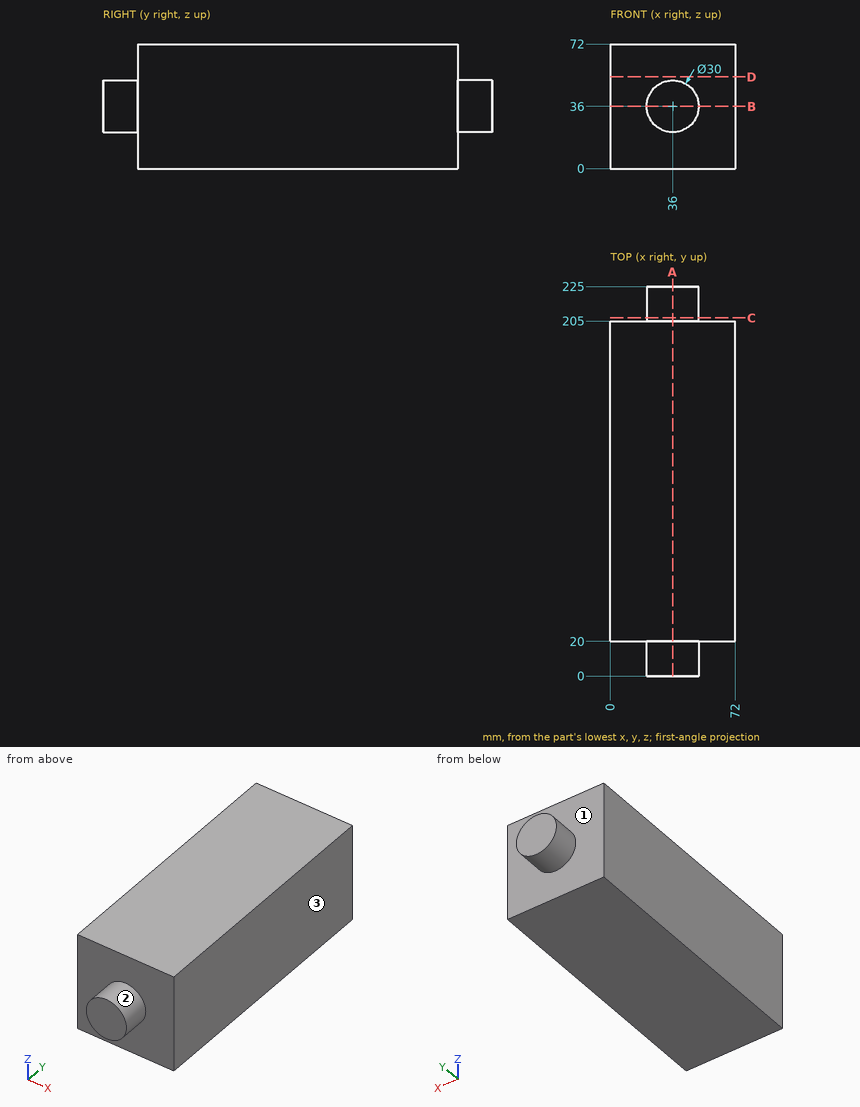
Job drawing, mm, ordinate dimensions from the low corner. One solid piece. A direction names the side the tool comes from. Give positions to 0.01 mm unless a question says otherwise; leave off trailing zeros. Loops run counter-clockwise (first coordinate to the right, second up) from the corner with the lowest first, then second, coordinate; pieces in that order, holes last. Notation, with made-up numbers: (18.25, 69) -> (74.25, 69) arc R29 ccw to (74.25, 100) -> close; hole circle Ø8 at (-12, 55.5). An arc over 180 degrees is marked (long way). Write each question's results on one line, items separated by ' | '.
(1) Flat gauge pins, fed straight in: pin 1 Ø1 at (x, z) = (48.5, 14.5) entering from +Y; pin 2 Ø8 at (x, z) = (55.5, 23.5) entering from -Y. Where does each tip first touch, or does it go through?
Geometry results:
pin 1: stops at y = 205 | pin 2: stops at y = 20
(2) Tool access for the marked faces 1, 2 and 3: list every direction of +Z, -Z, +X, -X, +Y, -Y with a clear straight run to the whole face (end or side of a thin tool).
Geometry results:
face 1: +Y | face 2: -Y | face 3: +Z, -Z, +X, +Y, -Y
(3) Cut at D-D on z = 53. List the corners of the cut face in (x, y).
Geometry results:
outline: (0, 20) -> (72, 20) -> (72, 205) -> (0, 205) -> close
(4) Cut at A-A on x = 36. List the corners of the cut face in (y, z), and give its area (3 significant figures).
Geometry results:
outline: (0, 21) -> (20, 21) -> (20, 0) -> (205, 0) -> (205, 21) -> (225, 21) -> (225, 51) -> (205, 51) -> (205, 72) -> (20, 72) -> (20, 51) -> (0, 51) -> close | area: 14,500 mm²
(5) Cut at C-C on y = 207. List the corners of the cut face in (x, z).
Geometry results:
outline: circle Ø30 at (36, 36)
(6) Probe line 1 along Y through (x, z) = (68, 57.5); line 2 along X through (y, z) = (14, 33.5). List the from-to ranges inside material, lowest first.
Geometry results:
line 1: y = 20 to 205 | line 2: x = 21.21 to 50.79
(7) Cut at B-B on z = 36. List the corners of the cut face in (x, y).
Geometry results:
outline: (0, 20) -> (21, 20) -> (21, 0) -> (51, 0) -> (51, 20) -> (72, 20) -> (72, 205) -> (51, 205) -> (51, 225) -> (21, 225) -> (21, 205) -> (0, 205) -> close
